Print and shaded views of the part. All mm, measured from the part's lowest x, y and z. A direction names the side the tool comes from. Round coordinates to 2 decimals unless told otherwise and drop trailing zeros. Loops run counter-clockwise (first coordinate to the right, second up) from the corner with the lowest first, then second, coordinate; pieces in that order, holes last. Notation, with made-up numbers: M 35,86 L 42,86 A32 ccw 42,116 Z; hole C 73,23.25 d3. An arc over 180 degrees is marked long. One line per item, written item: value. Start each with the question number.
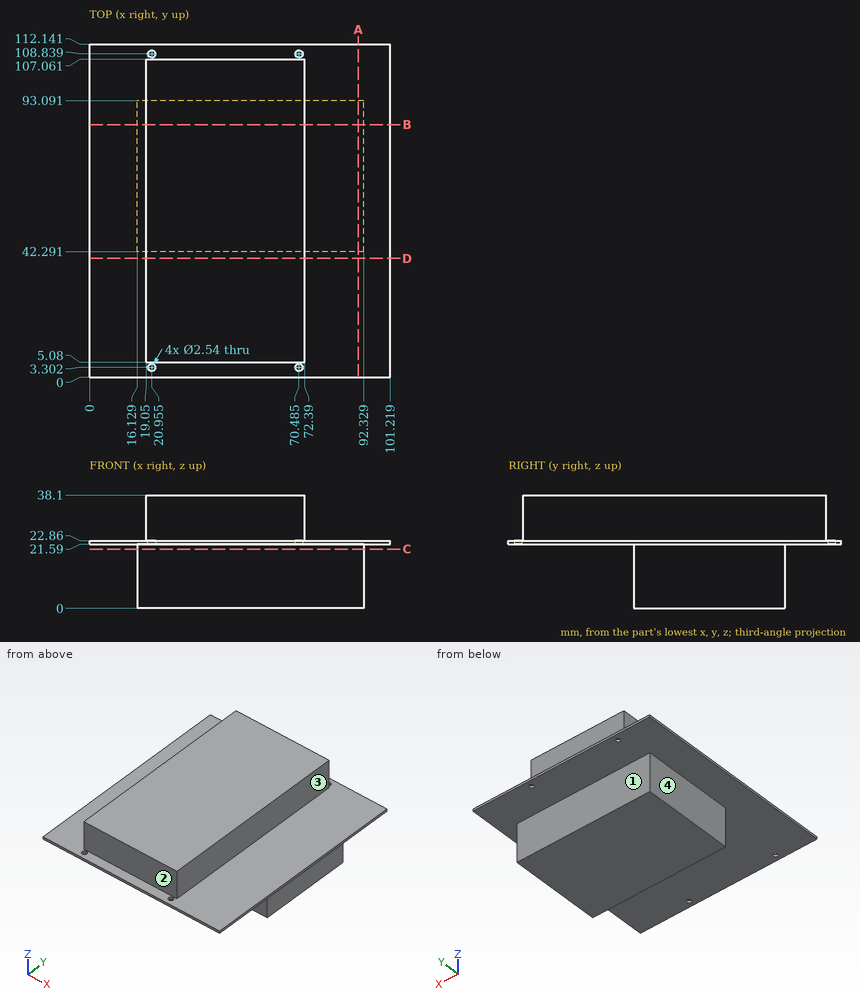
(1) Slice it at A-A, the plane x = 90.5. List the corners of the cut face in (y, z), and give its area (3 significant figures).
(2) Slice it at D-D, the plane y = 40. List the corners of the cut face in (x, z).
(3) Flat gauge pins, fed straight in: P1, Ø5, axis at y = 47, z = 30, coming from the -X side; P2, Ø4.5, axis at y = 46, z = 34, coming from the +X side; P3, Ø1, axis at x = 56.5, z = 18, coming from the +Y side; P4, Ø1.5, axis at x = 70.485, y = 3.302, coming from the +Z side. Where does each tip first touch, or does it go through?
(4) Which spindle directions (+Z, -Z, +X, -X, +Y, -Y) get a long thin tool onto all of the face, cutting with end or side? Do the marked faces 1, 2, 3 and 4. Say none if no direction does.
(5) Probe L1, parallel to Z at x = 14, y = 91.5; L2, parallel to Z at x = 41, y = 26; L3, parallel to X at y = 7, z = 36. List the from-to ranges inside material, lowest first.
(6) Slice it at B-B, the plane y = 85. List the corners of the cut face in (x, z).
(7) Slice it at C-C, the plane z = 20. List the corners of the cut face in (x, y).
Check result:
1. outline: M 0,21.59 L 42.29,21.59 L 42.29,0 L 93.09,0 L 93.09,21.59 L 112.14,21.59 L 112.14,22.86 L 0,22.86 Z
1. area: 1,240 mm^2
2. outline: M 0,21.59 L 101.22,21.59 L 101.22,22.86 L 72.39,22.86 L 72.39,38.1 L 19.05,38.1 L 19.05,22.86 L 0,22.86 Z
3. P1: stops at x = 19.05
3. P2: stops at x = 72.39
3. P3: stops at y = 93.09
3. P4: passes through
4. face 1: -Z, +X, -X, +Y
4. face 2: +Z, +X, -X, -Y
4. face 3: +Z, +X, +Y, -Y
4. face 4: -Z, -X, +Y, -Y
5. L1: z = 21.59 to 22.86
5. L2: z = 21.59 to 38.1
5. L3: x = 19.05 to 72.39
6. outline: M 0,21.59 L 16.13,21.59 L 16.13,0 L 92.33,0 L 92.33,21.59 L 101.22,21.59 L 101.22,22.86 L 72.39,22.86 L 72.39,38.1 L 19.05,38.1 L 19.05,22.86 L 0,22.86 Z
7. outline: M 16.13,42.29 L 92.33,42.29 L 92.33,93.09 L 16.13,93.09 Z
